Input: part model. Units: mm. Frame: model coordinates. Face numbers are marked on the shaded views. A direction names the side the tool comes from. Round coordinates to 2 decimals unless told otherwise and drop trailing zeros. Order: outer loops, then holes, each group sorted by start corner. A loop starts at its lowest first (then second) coordinate and runs counter-clockwise, first axis right, second up. Notation, with made-up numbers: (68.25, 20.25) -> (105.25, 20.25) arc R8 cw to (105.25, 32.25) -> close; hole circle Ø3 at (-35, 6). An arc over 180 degrees is marked (long way). Use a Markdown table: item, result.
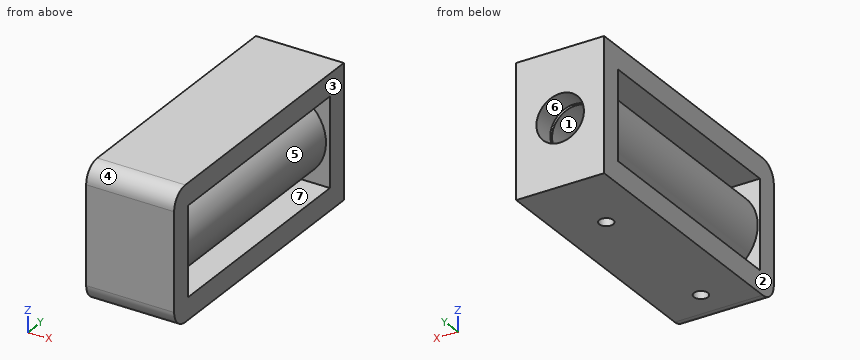
from build123d import *

# Parameters (mm, degrees)
SKETCH1_W           = 10
SKETCH1_H           = 15.08
BOSS_EXTRUDE1_DEPTH = 30.56
SKETCH2_W           = 10.08
SKETCH2_H           = 25.56
CUT_EXTRUDE1_DEPTH  = 20
SKETCH5_R           = 4.75
BOSS_EXTRUDE2_DEPTH = 25.25
SKETCH3_R           = 2.7
CUT_EXTRUDE2_DEPTH  = 20
FILLET1_R           = 2
CUT_EXTRUDE3_REACH  = 36.443
SKETCH4_R           = 0.8


with BuildPart() as part:
    # Sketch1 → Boss-Extrude1 (new body)
    with BuildSketch(Plane(origin=(0, 0, 0), x_dir=(1, 0, 0), z_dir=(0, 1, 0))):
        Rectangle(SKETCH1_W, SKETCH1_H)
    extrude(amount=BOSS_EXTRUDE1_DEPTH)

    # Sketch2 → Cut-Extrude1 (cut)
    with BuildSketch(Plane(origin=(5, 0, 0), x_dir=(0, 0, -1), z_dir=(1, 0, 0))):
        with Locations((0, 15.28)):
            Rectangle(SKETCH2_W, SKETCH2_H)
    extrude(amount=-CUT_EXTRUDE1_DEPTH, mode=Mode.SUBTRACT)

    # Sketch5 → Boss-Extrude2 (add)
    with BuildSketch(Plane(origin=(0, 2.5, 0), x_dir=(1, 0, 0), z_dir=(0, 1, 0))):
        with Locations(Location((0, 0, 0), (0, 0, 90))):
            Circle(SKETCH5_R)
    extrude(amount=BOSS_EXTRUDE2_DEPTH)

    # Sketch3 → Cut-Extrude2 (cut)
    with BuildSketch(Plane(origin=(0, 30.56, 0), x_dir=(1, 0, 0), z_dir=(0, 1, 0))):
        with Locations(Location((0, 0, 0), (0, 0, 270))):
            Circle(SKETCH3_R)
    extrude(amount=-CUT_EXTRUDE2_DEPTH, mode=Mode.SUBTRACT)

    # Fillet1
    fillet1_edges = [part.edges().sort_by_distance(p)[0] for p in [
        (0, 0, 7.54),
        (0, 0, -7.54),
    ]]
    fillet(fillet1_edges, radius=FILLET1_R)

    # Sketch4 → Cut-Extrude3 (cut, up to next)
    with BuildSketch(Plane(origin=(0, 0, -7.54), x_dir=(-1, 0, 0), z_dir=(0, 0, -1)), mode=Mode.PRIVATE) as cut_extrude3_sk1:
        with Locations((0, 22.26)):
            Circle(SKETCH4_R)
    cut_extrude3_tool1 = extrude(cut_extrude3_sk1.sketch, amount=-CUT_EXTRUDE3_REACH, mode=Mode.PRIVATE) & part.part
    # Sketch4 → Cut-Extrude3 (cut, up to next)
    with BuildSketch(Plane(origin=(0, 0, -7.54), x_dir=(-1, 0, 0), z_dir=(0, 0, -1)), mode=Mode.PRIVATE) as cut_extrude3_sk2:
        with Locations((0, 5.2)):
            Circle(SKETCH4_R)
    cut_extrude3_tool2 = extrude(cut_extrude3_sk2.sketch, amount=-CUT_EXTRUDE3_REACH, mode=Mode.PRIVATE) & part.part
    add(cut_extrude3_tool1.solids().sort_by_distance((0, 22.26, -7.54))[0], mode=Mode.SUBTRACT)
    add(cut_extrude3_tool2.solids().sort_by_distance((0, 5.2, -7.54))[0], mode=Mode.SUBTRACT)


solid = part.part
1) Pull-direction query (X, two-part tool) for the marked faces 1, 2, 3 and 4; classes: +X half, -X half, draft (parallel to the pull), parting line (faces both ways), or undercut.
Results found:
| item | result |
|---|---|
| face 1 | undercut |
| face 2 | -X half |
| face 3 | +X half |
| face 4 | draft |
2) Cut plane D-D on z = 0. Return loops of the section in (x, y).
Results found:
| item | result |
|---|---|
| outline | (-5, 0) -> (5, 0) -> (5, 2.5) -> (4.75, 2.5) -> (4.75, 27.75) -> (2.7, 27.75) -> (2.7, 10.56) -> (-2.7, 10.56) -> (-2.7, 27.75) -> (-4.75, 27.75) -> (-4.75, 2.5) -> (-5, 2.5) -> close; (-5, 28.06) -> (-2.7, 28.06) -> (-2.7, 30.56) -> (-5, 30.56) -> close; (2.7, 28.06) -> (5, 28.06) -> (5, 30.56) -> (2.7, 30.56) -> close |
3) Cut plane A-A on y = 22.26. Return loops of the section in (x, z).
Results found:
| item | result |
|---|---|
| outline | (-5, -7.54) -> (-0.8, -7.54) -> (-0.8, -5.04) -> (-5, -5.04) -> close; (-5, 5.04) -> (5, 5.04) -> (5, 7.54) -> (-5, 7.54) -> close; circle Ø9.5 at (0, 0); (0.8, -7.54) -> (5, -7.54) -> (5, -5.04) -> (0.8, -5.04) -> close; hole circle Ø5.4 at (0, 0) |
4) Cut plane C-C on y = 14. Return loops of the section in (x, z).
Results found:
| item | result |
|---|---|
| outline | (-5, -7.54) -> (5, -7.54) -> (5, -5.04) -> (-5, -5.04) -> close; (-5, 5.04) -> (5, 5.04) -> (5, 7.54) -> (-5, 7.54) -> close; circle Ø9.5 at (0, 0); hole circle Ø5.4 at (0, 0) |
5) Set-up query: the marked faces 5, 6 and 7. Return all of +Z, -Z, +X, -X, +Y, -Y with unobstructed straight access to the full face (end or side cutting, diameter ignored); none if empty.
Results found:
| item | result |
|---|---|
| face 5 | none |
| face 6 | +Y |
| face 7 | +X, -X |
6) Pin query (flat end, axial travel): pin 1 Ø5 at (y, z) = (12.5, 0.5) entering from -X. Return the tip coordinate at first contact, or that it passes through.
Results found:
| item | result |
|---|---|
| pin 1 | stops at x = -4.75 |
7) Line query: L1, parallel to X at y = 29.25, z = 0; L2, parallel to Z at x = -0.25, y = 3; L3, parallel to Z at x = 3.5, y = 18. Output: solid intervals per line, ascending. Write a range as [from, to].
Results found:
| item | result |
|---|---|
| L1 | x = [-5, -2.7], [2.7, 5] |
| L2 | z = [-7.54, -5.04], [-4.74, 4.74], [5.04, 7.54] |
| L3 | z = [-7.54, -5.04], [-3.21, 3.21], [5.04, 7.54] |
8) Cut plane B-B on x = 0. Count the separate pieces of the cut face and the enclosed holes in it, and give its area (3 significant figures).
Results found:
| item | result |
|---|---|
| separate pieces | 3 |
| enclosed holes | 0 |
| area | 327 mm² |
